```python
from build123d import *

# Parameters (mm, degrees)
SKETCH2_W           = 0.4
SKETCH2_H           = 1.95
BOSS_EXTRUDE1_DEPTH = 6


with BuildPart() as part:
    # Sketch1 → Revolve1 (revolve)
    with BuildSketch(Plane.XY):
        with BuildLine():
            Line((0, 0), (3, 0))
            Line((3, 0), (3, -3.4))
            Line((3, -3.4), (2.15, -3.4))
            Line((2.15, -3.4), (2.15, -6.2))
            Line((2.15, -6.2), (3.375, -6.2))
            Line((3.375, -6.2), (3.375, -12.8))
            Line((3.375, -12.8), (4.75, -12.8))
            Line((4.75, -12.8), (4.75, -14.35))
            ThreePointArc((4.75, -14.35), (4.389176995, -14.680340843), (3.914835346, -14.8))
            Line((3.914835346, -14.8), (3.4, -14.8))
            Line((3.4, -14.8), (3.4, -22))
            Line((3.4, -22), (0, -22))
            Line((0, -22), (0, 0))
        make_face()
    revolve(axis=Axis((0, -223.623157896, 0), (0, 1, 0)))

    # Sketch2 → Boss-Extrude1 (add)
    with BuildSketch(Plane.XZ.offset(22)):
        with Locations((-1.675, 0)):
            Rectangle(SKETCH2_W, SKETCH2_H)
        with Locations((1.675, 0)):
            Rectangle(SKETCH2_W, SKETCH2_H)
    extrude(amount=BOSS_EXTRUDE1_DEPTH)


solid = part.part
```
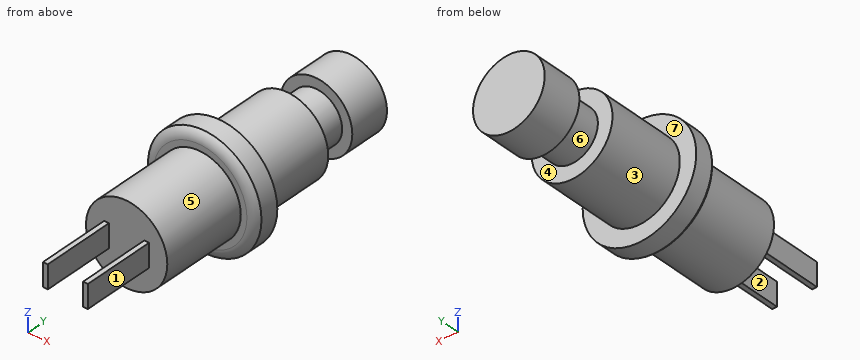
Can you work these out from the model? Positions are in its coordinate system, mm. Face numbers are marked on the shaded views. A direction names the side the tool comes from. Coordinates: 2 decimals unless noted, no trailing zeros. Loops run counter-clockwise (first coordinate to the right, second up) from the corner with the lowest first, then second, coordinate; pieces in that order, holes last.
1) I need wall thicknesses on probe 1 along X at (y, z) = (-5.25, 0); probe 2 along Y at (x, z) = (1.5, 2.5); probe 3 along Y at (x, z) = (-1.75, 3). Which ranges of each line are inside material? Lowest first, please.
2) Thinking about a two-plate mould opening in Y: for the marked faces 5, 6 and 7, which applies, pulls with the +Y half, pulls with the -Y half, needs draft (parallel to the pull), parting line crosses it, or undercut?
3) Imagine slicing it at A-A on x = 0. List the corners of the cut face in (y, z) for me (3 decimals).
4) For pin 1 (1 mm diameter, centred on y = -25.5, z = 0, fed in from -X) (3 decimals); pin 2 (1.6 mm diameter, centred on y = -26, z = 0, fed in from +X) (3 decimals); pin 3 (5 mm diameter, centred on x = 0, y = -3, fed in from +Z), each with a flat end and sliding along its axis, tell me the tip position at first contact or that it passes through.
5) Imagine slicing it at C-C on y = -20. List the corners of the cut face in (x, z) for me.
6) Which directions (+Z, -Z, +X, -X, +Y, -Y) give clear straight access to the entire face, cutting with the end or side of a thin tool? Please do the marked faces 1, 2, 3 and 4.
Completed:
1. probe 1: x = -2.15 to 2.15
1. probe 2: y = -22 to -6.2, -3.4 to 0
1. probe 3: y = -14.8 to -12.8
2. face 5: needs draft
2. face 6: undercut
2. face 7: pulls with the +Y half
3. outline: (-22, -3.4) - (-14.8, -3.4) - (-14.8, -3.915) arc R1 ccw to (-14.35, -4.75) - (-12.8, -4.75) - (-12.8, -3.375) - (-6.2, -3.375) - (-6.2, -2.15) - (-3.4, -2.15) - (-3.4, -3) - (0, -3) - (0, 3) - (-3.4, 3) - (-3.4, 2.15) - (-6.2, 2.15) - (-6.2, 3.375) - (-12.8, 3.375) - (-12.8, 4.75) - (-14.35, 4.75) arc R1 ccw to (-14.8, 3.915) - (-14.8, 3.4) - (-22, 3.4) - close
4. pin 1: stops at x = -1.875
4. pin 2: stops at x = 1.875
4. pin 3: stops at z = 3
5. outline: circle Ø6.8 at (0, 0)
6. face 1: +Z, -Z, +X, -Y
6. face 2: +Z, -Z, -Y
6. face 3: +Y
6. face 4: none
